```python
from build123d import *

# Parameters (mm, degrees)
F1_DEPTH = 78.74
F2_R     = 68.58
F3_DEPTH = 228.6
F4_W     = 81.28
F4_H     = 55.88
F5_DEPTH = 25.4


with BuildPart() as f1:
    # F0 (on Top) → F1 (new body)
    with BuildSketch(Plane.XY):
        Polygon((0, 0), (0, 38.1), (-21.834282, 44.45), (-59.849521, 41.91), (-76.2, 29.845), (-76.2, 0), align=None)
        Polygon((0, -38.1), (0, 0), (-76.2, 0), (-76.2, -29.845), (-59.849521, -41.91), (-21.834282, -44.45), align=None)
        Polygon((-76.2, -29.845), (-76.2, 0), (-76.2, 29.845), (-190.5, 29.845), (-215.9, 0), (-190.5, -29.845), align=None)
    extrude(amount=F1_DEPTH)

    # F2 (on face) → F3 (cut)
    with BuildSketch(Plane.YZ):
        Circle(F2_R)
    extrude(amount=-F3_DEPTH, mode=Mode.SUBTRACT)

    # F4 (on face) → F5 (cut)
    with BuildSketch(Plane.XY.offset(78.74)):
        with Locations((-121.92, 0)):
            Rectangle(F4_W, F4_H)
    extrude(amount=-F5_DEPTH, mode=Mode.SUBTRACT)


solid = f1.part
```
Geometry check sheet. Reference: the model listing, model coordinates, mm. A direction names the side the tool comes from. Give positions to 0.01 mm unless a question says otherwise; leave off trailing zeros. Order: outer loops, then holes, each group sorted by start corner. A loop starts at its lowest first (then second) coordinate and runs counter-clockwise, first axis right, second up. Notation, with made-up numbers: (85, 52.25) - (107, 52.25) arc R21 cw to (107, 78.25) - close; hole circle Ø3 at (41.5, 76.5). An arc over 180 degrees is marked (long way). Write item = value, one per line. Start each with the question number.
1) Section check C-C (y = -9). Enter the section's corners in (x, z).
2) Access from +Z, -Z, +X, -X, +Y, -Y to the whole of each face (thin tool, end or side, straight path). Record for faces 4 (the flat face through (-162.56, 0, 73)), 5 (the flat face through (-134, -29.845, 70)), 6 (the flat face through (0, -1, 73)).
3) Draft check along X on faces 1 (the flat face through (-203.022, 15.131, 72.012)), 2 (the flat face through (-81.28, 0, 73)), 3 (the flat face through (-133, 29.845, 70)). Enter one of: released by +X, released by -X, zero draft, split by the parting line, or undercut.
4) Section check D-D (z = 75.25). Enter the section's corners in (x, y) (3 decimals).
5) Scan lines: L1, parallel to Y at x = -115, z = 66 (3 decimals); L2, parallel to X at y = 13, z = 77.75; L3, parallel to Y at x = -42, z = 55. Record each from-to range of solid material in increasing order.
6) Section check B-B (z = 66.5). Enter the section's corners in (x, y) (3 decimals), then the cut area to 3 significant figures.
7) Section check A-A (x = -127). Enter the section's corners in (y, z) (3 decimals).
8) Gauge pin test, flat ends, axial feed: pin 1 Ø12 at (y, z) = (-27.5, 58) entering from -X; pin 2 Ø8 at (x, z) = (-139, 69) entering from -Y (3 decimals); pin 3 Ø13 at (y, z) = (7, 71) entering from -X. Record the tip position at first contact, or that the pin passes through.
Geometry check:
q1.outline = (-208.24, 67.99) - (-162.56, 67.99) - (-162.56, 78.74) - (-208.24, 78.74) - close; (-81.28, 67.99) - (0, 67.99) - (0, 78.74) - (-81.28, 78.74) - close
q2.face_4 = +Z, -Z
q2.face_5 = +Z, -Z, -X, -Y
q2.face_6 = +Z, -Z, +X, +Y, -Y
q3.face_1 = released by -X
q3.face_2 = undercut
q3.face_3 = zero draft
q4.outline = (-215.9, 0) - (-190.5, -29.845) - (-76.2, -29.845) - (-59.85, -41.91) - (-21.834, -44.45) - (0, -38.1) - (0, 38.1) - (-21.834, 44.45) - (-59.85, 41.91) - (-76.2, 29.845) - (-190.5, 29.845) - close; hole (-162.56, -27.94) - (-81.28, -27.94) - (-81.28, 27.94) - (-162.56, 27.94) - close
q5.L1 = -29.845 to -27.94, 27.94 to 29.845
q5.L2 = -204.84 to -162.56, -81.28 to 0
q5.L3 = -43.1 to -40.97, 40.97 to 43.1
q6.outline = (-201.634, -16.762) - (-190.5, -29.845) - (-76.2, -29.845) - (-59.85, -41.91) - (-21.834, -44.45) - (0, -38.1) - (0, -16.762) - (-81.28, -16.762) - (-81.28, -27.94) - (-162.56, -27.94) - (-162.56, -16.762) - close; (-201.634, 16.762) - (-162.56, 16.762) - (-162.56, 27.94) - (-81.28, 27.94) - (-81.28, 16.762) - (0, 16.762) - (0, 38.1) - (-21.834, 44.45) - (-59.85, 41.91) - (-76.2, 29.845) - (-190.5, 29.845) - close
q6.area = 5,020 mm2
q7.outline = (-29.845, 61.745) arc R68.58 cw to (-27.94, 62.63) - (-27.94, 78.74) - (-29.845, 78.74) - close; (27.94, 62.63) arc R68.58 cw to (29.845, 61.745) - (29.845, 78.74) - (27.94, 78.74) - close
q8.pin_1 = -194.19
q8.pin_2 = -29.845
q8.pin_3 = -215.47
